```python
from build123d import *

# Parameters (mm, degrees)
SKETCH_1_R      = 2.5
EXTRUDE_1_DEPTH = 2.5
SKETCH_2_R      = 2.5
EXTRUDE_2_DEPTH = 5


with BuildPart() as part:
    # 草图1 → 凸台-拉伸1 (new body, symmetric)
    with BuildSketch(Plane.XY):
        with BuildLine():
            Line((-4.5, -5), (-4.5, 5))
            ThreePointArc((-4.5, 5), (0, 9.5), (4.5, 5))
            Line((4.5, 5), (4.5, -5))
            ThreePointArc((4.5, -5), (0, -9.5), (-4.5, -5))
        make_face()
        with Locations((0, 5)):
            Circle(SKETCH_1_R, mode=Mode.SUBTRACT)
        with Locations((0, -5)):
            Circle(SKETCH_1_R, mode=Mode.SUBTRACT)
    extrude(amount=EXTRUDE_1_DEPTH, both=True)

    # 草图2 → 凸台-拉伸2 (add)
    with BuildSketch(Plane.XY.offset(2.5)):
        with BuildLine():
            Line((-39.402984594, -8.42217587), (35.597015406, 26.57782413))
            ThreePointArc((35.597015406, 26.57782413), (41.57782413, 24.402984594), (39.402984594, 18.42217587))
            Line((39.402984594, 18.42217587), (-35.597015406, -16.57782413))
            ThreePointArc((-35.597015406, -16.57782413), (-41.57782413, -14.402984594), (-39.402984594, -8.42217587))
        make_face()
        with Locations((-37.5, -12.5)):
            Circle(SKETCH_2_R, mode=Mode.SUBTRACT)
        with Locations((37.5, 22.5)):
            Circle(SKETCH_2_R, mode=Mode.SUBTRACT)
        with Locations((0, 5)):
            Circle(SKETCH_2_R, mode=Mode.SUBTRACT)
    extrude(amount=-EXTRUDE_2_DEPTH)


solid = part.part
```
Design review of the part built by this model. Coordinates are the model's own, in mm. A direction names the side the tool comes from. Coordinates: 2 decimals unless noted, no trailing zeros. Loops run counter-clockwise (first coordinate to the right, second up) from the corner with the lowest first, then second, coordinate; pieces in that order, holes last. Notation, with made-up numbers: (-39, 25) - (-12, 25) arc R13 cw to (-12, 43) - close; hole circle Ø1 at (34, -24.5). An arc over 180 degrees is marked (long way). Use CSV: the item, a comma, the result in double quotes. Start each with the question number.
1) The part is to be moulded in two halves that separate along Y. For faces 1 (the cylindrical face through (41.535, 24.492, 0.035)), 2 (the flat face through (-4.5, -4, 0)), 3 (the cylindrical face through (38.84, 24.61, 0.04)), say which applies: +Y half, -Y half, draft (parallel to the pull), parting line (faces both ways), or undercut.
2) Tool access review of faces 4 (the flat face through (-19.83, -9.22, 0.04)), 5 (the flat face through (4.5, -1, 0)), 6 (the cylindrical face through (-0.33, 7.48, -0.04)): name each direction out of +Z, -Z, +X, -X, +Y, -Y from which nothing blocks a thin tool from reaching the whole face with its end or side.
3) Wall thickness on L1, parallel to X at y = -4.5, z = 0.05; L2, parallel to Y at x = 0, z = 0.4; L3, parallel to X at y = -7, z = 1.4: over which ranges is each line inside the solid? List them lowest first. Write a range as from..to.
4) Consider section C-C on x = -37.5. Write out the cut boundary in (y, z), then the cut area to 3 significant figures.
5) For pin 1 Ø6 at (x, y) = (12.5, 20.5) entering from +Z; pin 2 Ø1 at (x, z) = (-1, 0.5) entering from +Y; pin 3 Ø0.9 at (y, z) = (-3.5, 0.5) entering from -X; pin 4 Ø2 at (y, z) = (3.5, -1.5) entering from +X, all flat-tipped, find the tip position at first contact; note any pin that passes through.
6) Consider section D-D on y = 10.5. Write out the cut boundary in (x, z).
7) Consider section B-B on y = 3.5. Write out the cut boundary in (x, z), then the cut area to 3 significant figures.
8) Consider section A-A on z = 0.5. Write out the cut boundary in (x, y).
Geometry says:
1,face 1,"parting line"
1,face 2,"draft"
1,face 3,"undercut"
2,face 4,"+Z, -Z, -Y"
2,face 5,"+Z, -Z, +X, -Y"
2,face 6,"+Z, -Z"
3,L1,"-31..-9.72, -4.5..-2.45, 2.45..4.5"
3,L2,"-9.5..-7.5, -2.5..2.5, 7.5..9.97"
3,L3,"-36.36..-15.07, -4.03..-1.5, 1.5..4.03"
4,outline,"(-17, -2.5) - (-15, -2.5) - (-15, 2.5) - (-17, 2.5) - close; (-10, -2.5) - (-7.53, -2.5) - (-7.53, 2.5) - (-10, 2.5) - close"
4,area,"22.3 mm^2"
5,pin 1,"through"
5,pin 2,"y = 9.73"
5,pin 3,"x = -29.82"
5,pin 4,"x = 9.57"
6,outline,"(1.14, -2.5) - (22.43, -2.5) - (22.43, 2.5) - (1.14, 2.5) - close"
7,outline,"(-13.86, -2.5) - (-2, -2.5) - (-2, 2.5) - (-13.86, 2.5) - close; (2, -2.5) - (7.43, -2.5) - (7.43, 2.5) - (2, 2.5) - close"
7,area,"86.4 mm^2"
8,outline,"(-39.4, -8.42) arc R4.5 ccw to (-35.6, -16.58) - (-4.5, -2.07) - (-4.5, -5) arc R4.5 ccw to (4.5, -5) - (4.5, 2.13) - (39.4, 18.42) arc R4.5 ccw to (35.6, 26.58) - close; hole circle Ø5 at (-37.5, -12.5); hole circle Ø5 at (0, -5); hole circle Ø5 at (0, 5); hole circle Ø5 at (37.5, 22.5)"
